For this review, take the finished solid that the model builds, in its own axes (mm). Face numbers are marked on the shaded views. A direction names the side the tool comes from. Coordinates: 2 decimals unless noted, no trailing zeros. Order: outer loops, then holes, each group sorted by start corner. A loop starts at its lowest first (then second) coordinate and runs counter-clockwise, first axis right, second up. Notation, with made-up numbers: (43, -30) -> (70, -30) arc R20 cw to (70, -6) -> close; hole circle Ø3 at (26.25, 74). An arc over 180 degrees is marked (long way). Return JSON: item names as keys, results as strings. Group by question number.
Item 1: Machinability: for the marked faces 1 and 2, which of the approach directions +Z, -Z, +X, -X, +Y, -Y give a long, thin tool a straight path to every point of the face, cutting with its end or side? Answer none if there is none.
Item 2: Draft analysis for pull direction Y (two halves, no side actions). For the marked faces 3, 4 and 5, state which applies: +Y half, -Y half, draft (parallel to the pull), parting line (faces both ways), or undercut.
Item 3: Take a section at D-D (x = -0.95). Write out the cut boundary in (y, z).
Item 4: Take a section at A-A (x = -0.3). Write out the cut boundary in (y, z).
Item 5: Insertion check: pin 1 (2 mm diameter, centred on x = 1.5, z = 8.5, fed in from +Y); pin 2 (1.5 mm diameter, centred on x = -1.5, y = 2, fed in from +Z); pin 3 (2 mm diameter, centred on x = -1, z = 11.5, fed in from -Y). Each pin has a flat end and moves straight along its axis. Give the tip position at first contact, or say it passes through.
Item 6: Take a section at B-B (y = 1.35). Write out the cut boundary in (x, z), then the cut area to 3 significant figures.
Item 7: For line 1 along Z through (x, y) = (1.5, 1.6); line 2 along Z through (x, y) = (0.8, 0.1); line 3 along X through (y, z) = (-0.5, 11.75), list the stretches that pass through material, from the lowest coordinate up.
Item 8: Take a section at C-C (z = 10.25). Write out the cut boundary in (x, y), then the cut area to 3 significant figures.
```python
from build123d import *

# Parameters (mm, degrees)
SKETCH_1_R          = 3
EXTRUDE_1_DEPTH     = 1
CUT_EXTRUDE_1_DEPTH = 1
SKETCH_3_R          = 1.5
EXTRUDE_2_DEPTH     = 12


with BuildPart() as part:
    # 草图1 → 凸台-拉伸1 (new body)
    with BuildSketch(Plane.XY):
        Circle(SKETCH_1_R)
    extrude(amount=EXTRUDE_1_DEPTH)

    # 草图2 → 切除-拉伸1 (cut)
    with BuildSketch(Plane(origin=(0, 0, 0), x_dir=(-1, 0, 0), z_dir=(0, 0, -1))):
        Polygon((1.154700538, 0), (0.577350269, 1), (-0.577350269, 1), (-1.154700538, 0), (-0.577350269, -1), (0.577350269, -1), align=None)
    extrude(amount=-CUT_EXTRUDE_1_DEPTH, mode=Mode.SUBTRACT)

    # 草图3 → 凸台-拉伸2 (add)
    with BuildSketch(Plane.XY.offset(1)):
        Circle(SKETCH_3_R)
    extrude(amount=EXTRUDE_2_DEPTH)


solid = part.part
```
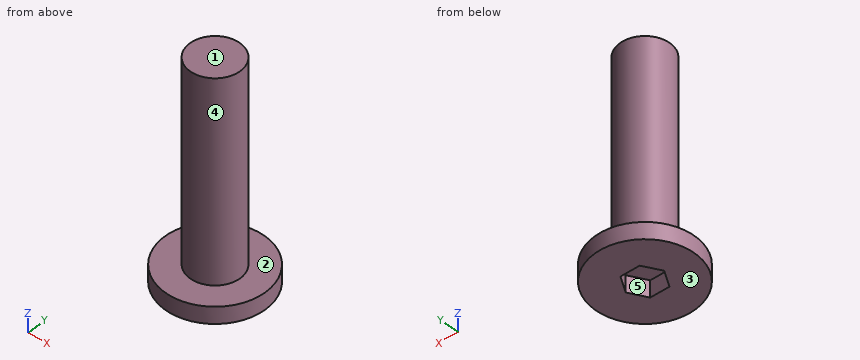
Findings below:
{
 "1": {"face 1": "+Z, +X, -X, +Y, -Y", "face 2": "+Z"},
 "2": {"face 3": "draft", "face 4": "parting line", "face 5": "undercut"},
 "3": {"outline": "(-2.85, 0) -> (-0.35, 0) -> (-0.35, 1) -> (0.35, 1) -> (0.35, 0) -> (2.85, 0) -> (2.85, 1) -> (1.16, 1) -> (1.16, 13) -> (-1.16, 13) -> (-1.16, 1) -> (-2.85, 1) -> close"},
 "4": {"outline": "(-2.98, 0) -> (-1, 0) -> (-1, 1) -> (1, 1) -> (1, 0) -> (2.98, 0) -> (2.98, 1) -> (1.47, 1) -> (1.47, 13) -> (-1.47, 13) -> (-1.47, 1) -> (-2.98, 1) -> close"},
 "5": {"pin 1": "stops at y = 1.41", "pin 2": "stops at z = 1", "pin 3": "stops at y = -1.5"},
 "6": {"outline": "(-2.68, 0) -> (2.68, 0) -> (2.68, 1) -> (0.65, 1) -> (0.65, 13) -> (-0.65, 13) -> (-0.65, 1) -> (-2.68, 1) -> close", "area": "21.1 mm2"},
 "7": {"line 1": "z = 0 to 1", "line 2": "z = 1 to 13", "line 3": "x = -1.41 to 1.41"},
 "8": {"outline": "circle Ø3 at (0, 0)", "area": "7.07 mm2"}
}
